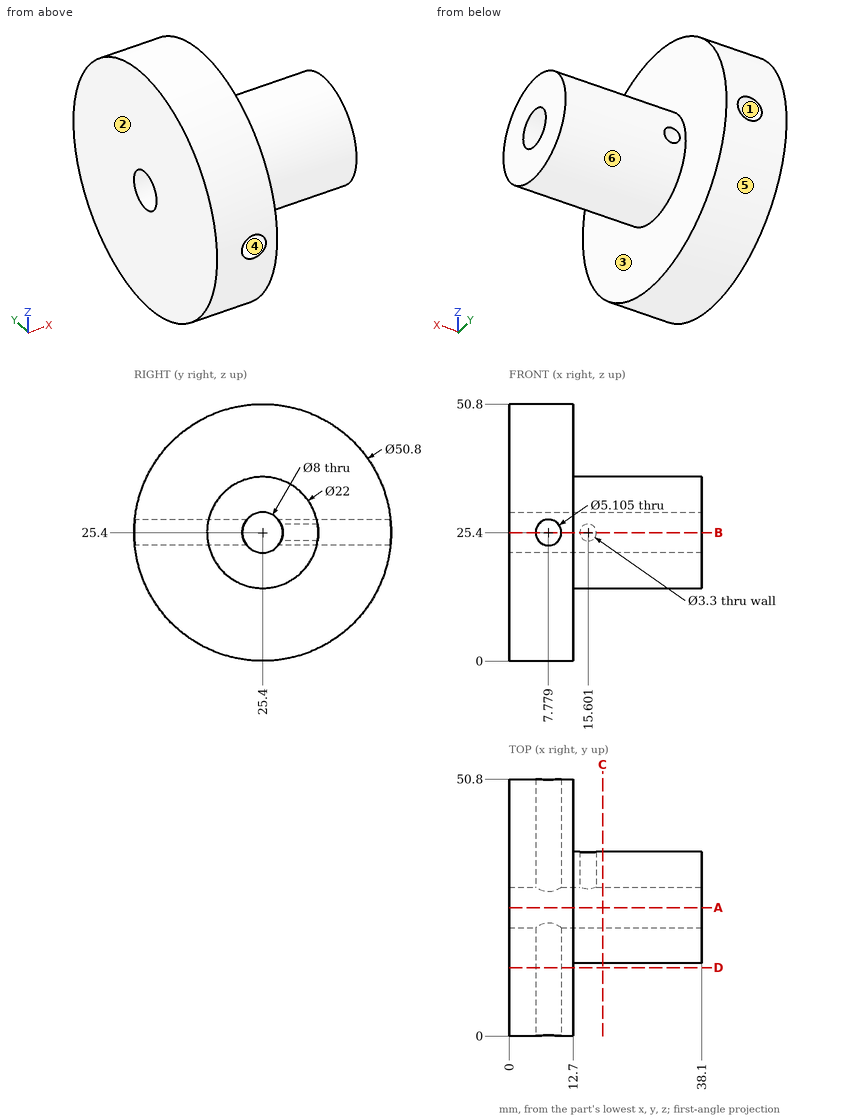
Check sheet for the drawn part. Datum: minimum x, y, z corner. Units: mm. A direction names the side the tool comes from. Coordinates: 2 decimals unless noted, no trailing zeros. Order: outer loops, then holes, each group sorted by start corner. A loop starts at its lowest first (then second) coordinate and runs counter-clockwise, first axis right, second up. Notation, with made-up numbers: (12, 75) -> (42, 75) arc R25 cw to (42, 91) -> close; hole circle Ø7 at (38, -15). An arc over 180 degrees is marked (long way). Use a Markdown table: item, result. Add a question column.
1. Go/stop test with flat-tipped pins: pin 1 Ø7 at (y, z) = (25.4, 25.4) entering from -X; pin 2 Ø2 at (x, z) = (15.6, 25.4) entering from +Y; pin 3 Ø8 at (x, z) = (27, 28.5) entering from -Y; pin 4 Ø8 at (x, y) = (15, 32.5) entering from -Z. Record where each tip stops, or that it passes through.
2. Mould release check, pull along X, two halves, no side actions. Record for the marked faces 1, 2, 3 and 4: pulls with the +X half, pulls with the -X half, needs draft (parallel to the pull), parting line crosses it, or undercut.
3. Cross-section at C-C (x = 18.5). Enter the section's corners in (y, z).
4. Material ranges on L1, parallel to X at y = 10.75, z = 25.4; L2, parallel to X at y = 34, z = 25; L3, parallel to X at y = 35, z = 25.4, recorded low to high.
5. Cross-section at A-A (y = 25.4). Enter the section's corners in (x, z).
6. Cross-section at D-D (y = 13.5). Enter the section's corners in (x, z) (1 decimal).
7. Set-up check for the marked faces 5 and 6: record each of +Z, -Z, +X, -X, +Y, -Y from which the full face is reachable in a straight line by a thin tool's end or side.
8. Cross-section at B-B (z = 25.4). Enter the section's corners in (x, y).
Filled sheet:
| question | item | result |
|---|---|---|
| 1 | pin 1 | through |
| 1 | pin 2 | y = 21.53 |
| 1 | pin 3 | y = 14.4 |
| 1 | pin 4 | z = 0.29 |
| 2 | face 1 | undercut |
| 2 | face 2 | pulls with the -X half |
| 2 | face 3 | pulls with the +X half |
| 2 | face 4 | undercut |
| 3 | outline | circle Ø22 at (25.4, 25.4); hole circle Ø8 at (25.4, 25.4) |
| 4 | L1 | 0 to 5.23, 10.33 to 12.7 |
| 4 | L2 | 0 to 5.26, 10.3 to 14, 17.2 to 38.1 |
| 4 | L3 | 0 to 5.23, 10.33 to 13.95, 17.25 to 38.1 |
| 5 | outline | (0, 0) -> (12.7, 0) -> (12.7, 14.4) -> (38.1, 14.4) -> (38.1, 21.4) -> (0, 21.4) -> close; (0, 29.4) -> (38.1, 29.4) -> (38.1, 36.4) -> (12.7, 36.4) -> (12.7, 50.8) -> (0, 50.8) -> close |
| 6 | outline | (0, 3) -> (12.7, 3) -> (12.7, 47.8) -> (0, 47.8) -> close; hole circle Ø5.1 at (7.8, 25.4) |
| 7 | face 5 | +X, -X |
| 7 | face 6 | +X |
| 8 | outline | (0, 0) -> (5.23, 0) -> (5.23, 21.4) -> (0, 21.4) -> close; (0, 29.4) -> (5.23, 29.4) -> (5.23, 50.8) -> (0, 50.8) -> close; (10.33, 0) -> (12.7, 0) -> (12.7, 14.4) -> (38.1, 14.4) -> (38.1, 21.4) -> (10.33, 21.4) -> close; (10.33, 29.4) -> (13.95, 29.4) -> (13.95, 36.4) -> (12.7, 36.4) -> (12.7, 50.8) -> (10.33, 50.8) -> close; (17.25, 29.4) -> (38.1, 29.4) -> (38.1, 36.4) -> (17.25, 36.4) -> close |
